Model file for the job. Use its own axes, mm. Face numbers are marked on the shaded views. A direction names the side the tool comes from. Round coordinates to 2 decimals unless told otherwise and drop trailing zeros. Order: outer loops, then holes, each group sorted by start corner. A loop starts at its lowest first (then second) coordinate and runs counter-clockwise, first axis right, second up. Notation, with made-up numbers: (75, -39) -> (117, -39) arc R24 cw to (117, -15) -> close; hole circle Ø2 at (14, 73). An arc over 180 degrees is marked (long way). Put each result on its own line as item: value. Start each with the question number.
Q1. Probe L1, parallel to Z at x = 72.5, y = 23; L2, parallel to X at y = 18, z = -4; L3, parallel to Z at x = 109, y = 19. List the from-to ranges inside material, lowest first.
Q2. Cut at C-C, the plane y = 13. List the corners of the cut face in (x, z), and give its area (3 significant figures).
Q3. Flat gauge pins, fed straight in: P1, Ø3, axis at y = 26.5, z = -55, coming from the +X side; P2, Ø5, axis at x = 15, y = 3.5, coming from the +Z side; P3, Ø7, axis at y = 17, z = 5.5, coming from the +X side. Where does each tip first touch, or does it go through?
Q4. 3-axis set-ups, long thin cutter, end or side, ignore diameter. For the marked faces 1, 2, 3 and 4: which of +Z, -Z, +X, -X, +Y, -Y reach the whole face in a straight line?
Q5. Cut at B-B, the plane y = 28. List the corners of the cut face in (x, z), and give its area (3 significant figures).
Q6. Cut at A-A, the plane x = 72. List the corners of the cut face in (y, z), and give its area (3 significant figures).
from build123d import *

# Parameters (mm, degrees)
SKETCH_1_W          = 116
SKETCH_1_H          = 69
EXTRUDE_1_DEPTH     = 32
SKETCH_2_W          = 7.5
SKETCH_2_H          = 66
CUT_EXTRUDE_1_DEPTH = 22
SKETCH_3_W          = 84
SKETCH_3_H          = 11
EXTRUDE_2_DEPTH     = 9


with BuildPart() as part:
    # 草图1 → 凸台-拉伸1 (new body)
    with BuildSketch(Plane(origin=(0, 0, 0), x_dir=(1, 0, 0), z_dir=(0, 1, 0))):
        with Locations((58, 34.5)):
            Rectangle(SKETCH_1_W, SKETCH_1_H)
    extrude(amount=EXTRUDE_1_DEPTH)

    # 草图2 → 切除-拉伸1 (cut)
    with BuildSketch(Plane(origin=(0, 32, 0), x_dir=(1, 0, 0), z_dir=(0, 1, 0))):
        with Locations((112.25, 33)):
            Rectangle(SKETCH_2_W, SKETCH_2_H)
        with Locations((3.75, 33)):
            Rectangle(SKETCH_2_W, SKETCH_2_H)
    extrude(amount=-CUT_EXTRUDE_1_DEPTH, mode=Mode.SUBTRACT)

    # 草图3 → 凸台-拉伸2 (add)
    with BuildSketch(Plane.XY):
        with Locations((55.5, 15.5)):
            Rectangle(SKETCH_3_W, SKETCH_3_H)
    extrude(amount=EXTRUDE_2_DEPTH)


solid = part.part
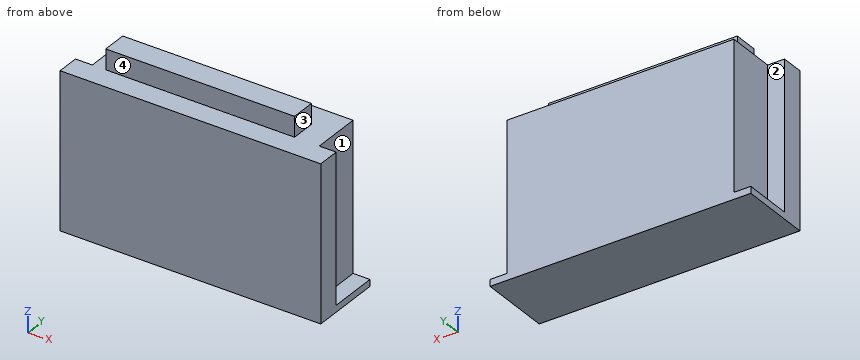
Ans:
1. L1: z = -69 to 0
1. L2: x = 7.5 to 108.5
1. L3: z = -69 to -66
2. outline: (0, -69) -> (116, -69) -> (116, -66) -> (108.5, -66) -> (108.5, 0) -> (97.5, 0) -> (97.5, 9) -> (13.5, 9) -> (13.5, 0) -> (7.5, 0) -> (7.5, -66) -> (0, -66) -> close
2. area: 7,770 mm^2
3. P1: stops at x = 108.5
3. P2: stops at z = 0
3. P3: stops at x = 97.5
4. face 1: +Z, +X, +Y
4. face 2: +Z, -X, +Y
4. face 3: +Z, +X, +Y, -Y
4. face 4: +Z, +X, -X, -Y
5. outline: (0, -69) -> (116, -69) -> (116, -66) -> (108.5, -66) -> (108.5, 0) -> (7.5, 0) -> (7.5, -66) -> (0, -66) -> close
5. area: 7,010 mm^2
6. outline: (0, -69) -> (32, -69) -> (32, 0) -> (21, 0) -> (21, 9) -> (10, 9) -> (10, 0) -> (0, 0) -> close
6. area: 2,310 mm^2
